CAD build for the part. Positions are in the model's coordinates, mm. Coordinates: 2 decimals unless noted, no trailing zeros. Loops run counter-clockwise (first coordinate to the right, second up) from the corner with the lowest first, then second, coordinate; pieces in that order, holes last.
1) Saw through at A-A, the plane y = 78.5. Write the cut outline in (x, z), and give its area (3 significant figures).
2) Two-plate mould, pull along Z, no slides. Class faces 1 (the flat face through (3.13, 92.79, -53.29)), 2 (the flat face through (3.13, 92.54, 53.72)), 3 (the cylindrical face through (3.131, -30.927, -55.247)): +Z half, -Z half, draft (parallel to the pull), parting line (faces both ways), or undercut.
3) Pin check, flat tips, straight feed: pin 1 Ø1.5 at (x, z) = (3, 10) entering from +Y; pin 2 Ø3 at (x, z) = (3, 30) entering from +Y. Stop position of each tip, or through.
4) Wall check: line 1 along Y through (x, z) = (2.75, 0); line 2 along Y through (x, z) = (6.25, -2); line 3 along Y through (x, z) = (6, 88.5). Give the ranges that are in metal, low to high.
5) Saw through at C-C, the plane y = 50.75. Write the cut outline in (x, z).
```python
from build123d import *

# Parameters (mm, degrees)
SKETCH1_R                        = 11.110595
BOSS_EXTRUDE1_DEPTH              = 6.35
F_11_64_0_17188_DIAMETER_HOLE1_D = 4.365752
CIRPATTERN1_COUNT                = 3


with BuildPart() as part:
    # Sketch1 → Boss-Extrude1 (new body)
    with BuildSketch(Plane(origin=(0, 0, 0), x_dir=(0, 0, -1), z_dir=(1, 0, 0))):
        with BuildLine():
            Line((38.200000054, 101.5), (68.801578457, 83.832170471))
            ThreePointArc((68.801578457, 83.832170471), (54.819408013, 31.649999973), (107.001578511, 17.667829529))
            Line((107.001578511, 17.667829529), (107.001578511, -17.667829529))
            ThreePointArc((107.001578511, -17.667829529), (54.819408013, -31.649999973), (68.801578457, -83.832170471))
            Line((68.801578457, -83.832170471), (38.200000054, -101.5))
            ThreePointArc((38.200000054, -101.5), (0, -63.299999946), (-38.200000054, -101.5))
            Line((-38.200000054, -101.5), (-68.801578457, -83.832170471))
            ThreePointArc((-68.801578457, -83.832170471), (-54.819408013, -31.649999973), (-107.001578511, -17.667829529))
            Line((-107.001578511, -17.667829529), (-107.001578511, 17.667829529))
            ThreePointArc((-107.001578511, 17.667829529), (-54.819408013, 31.649999973), (-68.801578457, 83.832170471))
            Line((-68.801578457, 83.832170471), (-38.200000054, 101.5))
            ThreePointArc((-38.200000054, 101.5), (0, 63.299999946), (38.200000054, 101.5))
        make_face()
        Circle(SKETCH1_R, mode=Mode.SUBTRACT)
    extrude(amount=BOSS_EXTRUDE1_DEPTH)

    # 11/64 (0.17188) Diameter Hole1 (through all)
    with Locations(Plane(origin=(6.35, 0, 0), x_dir=(0, 0, -1), z_dir=(1, 0, 0))):
        with Locations((0, 25.4)):
            f_11_64_0_17188_diameter_hole1 = Hole(F_11_64_0_17188_DIAMETER_HOLE1_D / 2)

    # CirPattern1: 11/64 (0.17188) Diameter Hole1 ×3 about axis
    cirpattern1_axis = Axis((0, 0, 0), (1, 0, 0))
    for i in range(1, CIRPATTERN1_COUNT):
        add(f_11_64_0_17188_diameter_hole1.rotate(cirpattern1_axis, i * 360 / CIRPATTERN1_COUNT), mode=Mode.SUBTRACT)


solid = part.part
```
Data:
1. outline: (0, -61.65) - (6.35, -61.65) - (6.35, -30.5) - (0, -30.5) - close; (0, 30.5) - (6.35, 30.5) - (6.35, 61.65) - (0, 61.65) - close
1. area: 396 mm2
2. face 1: -Z half
2. face 2: +Z half
2. face 3: undercut
3. pin 1: stops at y = 64.84
3. pin 2: stops at y = 79.89
4. line 1: y = -63.3 to -11.11, 11.11 to 23.22, 27.58 to 63.3
4. line 2: y = -63.35 to -10.93, 10.93 to 24.53, 26.27 to 63.35
4. line 3: y = -12.55 to 12.55
5. outline: (0, -49.7) - (6.35, -49.7) - (6.35, 49.7) - (0, 49.7) - close
